Build history of the part. All positions in model axes, mm. Round coordinates to 2 decimals unless told otherwise and drop trailing zeros. Order: outer loops, then holes, each group sorted by start corner. A loop starts at its lowest first (then second) coordinate and runs counter-clockwise, first axis right, second up. Notation, with made-up numbers: M 35,8.25 L 39,8.25 A25 cw 39,27.25 Z; hole C 69.5,-19 d6. An arc over 180 degrees is marked long. Use CSV: the item, a comma, the result in double quotes.
Autodesk Inventor part; units mm, degrees
ref_plane "YZ Plane" through (0, 0, 0) normal (1, 0, 0) x (0, 1, 0)
ref_plane "XZ Plane" through (0, 0, 0) normal (0, 1, 0) x (-1, 0, 0)
ref_plane "XY Plane" through (0, 0, 0) normal (0, 0, 1) x (1, 0, 0)
sketch "Sketch1" plane through (0, 0, 0) normal (0, 0, 1) x (1, 0, 0)
  circle A0 centre (0, 0) radius 10.5
  circle A1 centre (0, 0) radius 13 construction
  line L0 (7.8722, 12.365) -> (14.6445, 0.635)
  line L1 (14.6445, -0.635) -> (7.8722, -12.365)
  line L2 (6.7723, -13) -> (-6.7723, -13)
  line L3 (-7.8722, -12.365) -> (-14.6445, -0.635)
  line L4 (-14.6445, 0.635) -> (-7.8722, 12.365)
  line L5 (-6.7723, 13) -> (6.7723, 13)
  arc A2 (-6.7723, 13) -> (-7.8722, 12.365) centre (-6.7723, 11.73) ccw
  arc A3 (-14.6445, 0.635) -> (-14.6445, -0.635) centre (-13.5446, 0) ccw
  arc A4 (-7.8722, -12.365) -> (-6.7723, -13) centre (-6.7723, -11.73) ccw
  arc A5 (6.7723, -13) -> (7.8722, -12.365) centre (6.7723, -11.73) ccw
  arc A6 (14.6445, -0.635) -> (14.6445, 0.635) centre (13.5446, 0) ccw
  arc A7 (7.8722, 12.365) -> (6.7723, 13) centre (6.7723, 11.73) ccw
  point P0 (0, 13)
  point P1 (7.5056, 13)
  point P2 (15.0111, 0)
  point P3 (7.5056, -13)
  point P4 (-7.5056, -13)
  point P5 (-15.0111, 0)
  point P6 (-7.5056, 13)
  dimension "d1" = 26
  dimension "d0" = 21
  dimension "d2" = 1.27
extrude "Extrusion1" add sketch "Sketch1" along normal blind 3.81
properties part number "connector_nut" material "Lead"
(1) Drop flat-ended pins along their axis: pin 1 (1.5 mm diameter, centred on y = 6.5, z = 0.5, fed in from +X); pin 2 (6 mm diameter, centred on x = -2.5, y = -7, fed in from -Z); pin 3 (1 mm diameter, centred on x = 11, z = 1.5, fed in from +Y); pin 4 (2 mm diameter, centred on y = 6.5, z = 3.5, fed in from +X). Give the stop position or say it passes through.
Answer block:
pin 1,"stops at x = 11.69"
pin 2,"passes through"
pin 3,"stops at y = 7.81"
pin 4,"stops at x = 11.84"
(2) Two-plate mould, pull along X, no slides. Class faces 1 (the face through (14.815, 0.009, 1.878)), 2 (the face through (-14.815, -0.009, 1.878)), 3 (the face through (10, -3.2, 1.9)), 4 (the face through (0, -13, 2)): released by +X, released by -X, zero draft, split by the parting line, or undercut.
Answer block:
face 1,"released by +X"
face 2,"released by -X"
face 3,"undercut"
face 4,"zero draft"
(3) Cut at B-B, the plane y = 0. Give the cut face in (x, z), and give its area (3 significant figures).
Answer block:
outline,"M -14.81,0 L -10.5,0 L -10.5,3.81 L -14.81,3.81 Z; M 10.5,0 L 14.81,0 L 14.81,3.81 L 10.5,3.81 Z"
area,"32.9 mm²"
(4) Cut at C-C, the plane z = 0.65. Give the cut face in (x, y) (1 decimal).
Answer block:
outline,"M -14.6,-0.6 L -7.9,-12.4 A1.3 ccw -6.8,-13 L 6.8,-13 A1.3 ccw 7.9,-12.4 L 14.6,-0.6 A1.3 ccw 14.6,0.6 L 7.9,12.4 A1.3 ccw 6.8,13 L -6.8,13 A1.3 ccw -7.9,12.4 L -14.6,0.6 A1.3 ccw Z; hole C 0,0 d21"
(5) Cut at D-D, the plane y = -11. Give the cut face in (x, z).
Answer block:
outline,"M -8.66,0 L 8.66,0 L 8.66,3.81 L -8.66,3.81 Z"
(6) Cut at A-A, the plane x = 0. Give the cut face in (y, z).
Answer block:
outline,"M -13,0 L -10.5,0 L -10.5,3.81 L -13,3.81 Z; M 10.5,0 L 13,0 L 13,3.81 L 10.5,3.81 Z"
(7) Wall check: line 1 (Y direction, x = 0, z = 1.4); line 2 (X direction, y = 5.75, z = 1.9); line 3 (X direction, y = 7.75, z = 2.8). Give the ranges that are in metal, low to high. Write a range as from..to.
Answer block:
line 1,"y = -13..-10.5, 10.5..13"
line 2,"x = -11.69..-8.79, 8.79..11.69"
line 3,"x = -10.54..-7.08, 7.08..10.54"
